Can you work these out from the model? Positions are in its coordinate system, mm. A direction names the side the tool comes from. Round coordinates to 2 decimals unless told otherwise and drop trailing zeros. Loops run counter-clockwise (first coordinate to the right, second up) from the corner with the lowest first, then second, coordinate; pieces in that order, holes last. Notation, with made-up numbers: M -22,35 L 35,35 A10 cw 35,41 Z; hole C 74.25,-31.75 d11. An arc over 180 degrees is marked long. Use a Markdown table: item, result. Add a question column.
Autodesk Fusion 360 part; units mm, degrees
sketch "Sketch1" plane through (0, 0, 0) normal (0, 0, 1) x (1, 0, 0)
  line L0 (-25, 25) -> (25, 25) construction
  line L1 (25, 25) -> (25, -25) construction
  line L2 (25, -25) -> (-25, -25) construction
  line L3 (-25, -25) -> (-25, 25) construction
  line L4 (-25, 25) -> (25, -25) construction
  line L5 (25, 25) -> (-25, -25) construction
  line L6 (24, 24) -> (-24, 24) construction
  line L7 (-24, 24) -> (-24, -24) construction
  line L8 (-24, -24) -> (24, -24) construction
  line L9 (24, -24) -> (24, 24) construction
  line L10 (24, 24) -> (-24, -24) construction
  line L11 (-24, 24) -> (24, -24) construction
  circle A0 centre (-22.5, 22.5) radius 1.5
  line L12 (0, 24) -> (0, -24)
  line L13 (-24, 0) -> (24, 0)
  circle A1 centre (-22.5, 22.5) radius 2.5 construction
  line L14 (-25, 0) -> (-25, 22.5)
  line L15 (0, 25) -> (-22.5, 25)
  arc A2 (-22.5, 25) -> (-25, 22.5) centre (-22.5, 22.5) ccw
  circle A3 centre (22.5, 22.5) radius 1.5
  arc A4 (25, 22.5) -> (22.5, 25) centre (22.5, 22.5) ccw
  line L16 (25, 0) -> (25, 22.5)
  line L17 (0, 25) -> (22.5, 25)
  circle A5 centre (-22.5, -22.5) radius 1.5
  arc A6 (-25, -22.5) -> (-22.5, -25) centre (-22.5, -22.5) ccw
  arc A7 (22.5, -25) -> (25, -22.5) centre (22.5, -22.5) ccw
  line L18 (25, 0) -> (25, -22.5)
  line L19 (0, -25) -> (-22.5, -25)
  line L20 (0, -25) -> (22.5, -25)
  line L21 (-25, 0) -> (-25, -22.5)
  circle A8 centre (22.5, -22.5) radius 1.5
  dimension "d1" = 50
  dimension "d2" = 50
  dimension "d3" = 48
  dimension "d4" = 48
  dimension "d5" = 1.5
extrude "Extrude1" add sketch "Sketch1" along normal blind 3
sketch "Sketch2" plane through (0, 0, 3) normal (0, 0, 1) x (-1, 0, 0)
  circle A0 centre (22.5, -22.5) radius 1.5
  circle A1 centre (-22.5, -22.5) radius 1.5
  circle A2 centre (-22.5, 22.5) radius 1.5
  circle A3 centre (22.5, 22.5) radius 1.5
  line L0 (-22.5, -25) -> (22.5, -25)
  arc A4 (22.5, -25) -> (25, -22.5) centre (22.5, -22.5) ccw
  line L1 (25, -22.5) -> (25, 22.5)
  arc A5 (25, 22.5) -> (22.5, 25) centre (22.5, 22.5) ccw
  line L2 (22.5, 25) -> (-22.5, 25)
  arc A6 (-22.5, 25) -> (-25, 22.5) centre (-22.5, 22.5) ccw
  line L3 (-25, 22.5) -> (-25, -22.5)
  arc A7 (-25, -22.5) -> (-22.5, -25) centre (-22.5, -22.5) ccw
  line L4 (18, 20) -> (10, 20)
  line L5 (10, 20) -> (10, 27)
  line L6 (10, 27) -> (18, 27)
  line L7 (18, 27) -> (18, 20)
  line L8 (8.1443, 19.89) -> (1.4935, 19.89)
  line L9 (1.4935, 19.89) -> (1.4935, 25)
  line L10 (1.4935, 25) -> (8.1443, 25)
  line L11 (8.1443, 25) -> (8.1443, 19.89)
  line L12 (-6.1327, 6.202) -> (-13.0241, 6.202)
  line L13 (-13.0241, 6.202) -> (-13.0241, 13.2304)
  line L14 (-13.0241, 13.2304) -> (-6.1327, 13.2304)
  line L15 (-6.1327, 13.2304) -> (-6.1327, 6.202)
  line L16 (9.0194, 12.5915) -> (1.9406, 12.5915)
  line L17 (1.9406, 12.5915) -> (1.9406, 3.3668)
  line L18 (1.9406, 3.3668) -> (9.0194, 3.3668)
  line L19 (9.0194, 3.3668) -> (9.0194, 12.5915)
  line L20 (18.1054, 2.8016) -> (12.2514, 2.8016)
  line L21 (12.2514, 2.8016) -> (12.2514, 8.8879)
  line L22 (12.2514, 8.8879) -> (18.1054, 8.8879)
  line L23 (18.1054, 8.8879) -> (18.1054, 2.8016)
  line L24 (23.1634, -18.1139) -> (7.6017, -18.1139)
  line L25 (7.6017, -18.1139) -> (7.6017, -12.2414)
  line L26 (7.6017, -12.2414) -> (23.1634, -12.2414)
  line L27 (23.1634, -12.2414) -> (23.1634, -18.1139)
  line L28 (-1.1153, -18.1139) -> (-17.3248, -18.1139)
  line L29 (-17.3248, -18.1139) -> (-17.3248, -12.2845)
  line L30 (-17.3248, -12.2845) -> (-1.1153, -12.2845)
  line L31 (-1.1153, -12.2845) -> (-1.1153, -18.1139)
  line L32 (17.5, -21) -> (9.5, -21)
  line L33 (9.5, -21) -> (9.5, -29)
  line L34 (9.5, -29) -> (17.5, -29)
  line L35 (17.5, -29) -> (17.5, -21)
  line L36 (-4, -21) -> (-12, -21)
  line L37 (-12, -21) -> (-12, -29)
  line L38 (-12, -29) -> (-4, -29)
  line L39 (-4, -29) -> (-4, -21)
  line L40 (-21.1194, -13.1989) -> (-25, -13.1989)
  line L41 (-25, -13.1989) -> (-25, -6.7401)
  line L42 (-25, -6.7401) -> (-21.1194, -6.7401)
  line L43 (-21.1194, -6.7401) -> (-21.1194, -13.1989)
  line L44 (-17, -0.5) -> (-33, -0.5)
  line L45 (-33, -0.5) -> (-33, 5.5)
  line L46 (-33, 5.5) -> (-17, 5.5)
  line L47 (-17, 5.5) -> (-17, -0.5)
  dimension "d8" = 2
  dimension "d9" = 7
  dimension "d10" = 8
  dimension "d11" = 7
  dimension "d12" = 4
  dimension "d13" = 8
  dimension "d14" = 8
  dimension "d15" = 8
  dimension "d16" = 7.5
  dimension "d17" = 13
  dimension "d18" = 8
  dimension "d19" = 6
  dimension "d20" = 16
  dimension "d21" = 19.5
extrude "Extrude2" add sketch "Sketch2" along normal blind 8 contours L3 L44 L45 L46 | L3 L44 L46 L47
extrude "Extrude3" add sketch "Sketch2" along normal blind 5 contours L0 L36 L37 L39 | L0 L37 L38 L39 | L0 L32 L33 L35 | L0 L33 L34 L35
extrude "Extrude4" add sketch "Sketch2" along normal blind 3 contours L3 L40 L41 L42 L43 | L2 L8 L9 L10 L11 | L2 L4 L5 L7 | L2 L5 L6 L7
extrude "Extrude5" add sketch "Sketch2" along normal blind 2 contours L16 L17 L18 L19
extrude "Extrude6" add sketch "Sketch2" along normal blind 1.5 contours L12 L13 L14 L15 | L20 L21 L22 L23 | L24 L25 L26 L27 | L28 L29 L30 L31
sketch "Sketch3" plane through (0, 0, 3) normal (0, 0, 1) x (-1, 0, 0)
  line L0 (-1.1153, -12.2845) -> (-1.1153, -18.1139)
  line L1 (-1.1153, -18.1139) -> (-17.3248, -18.1139)
  line L2 (-17.3248, -18.1139) -> (-17.3248, -12.2845)
  line L3 (-17.3248, -12.2845) -> (-1.1153, -12.2845)
  line L4 (-6.1327, 13.2304) -> (-6.1327, 6.202)
  line L5 (-6.1327, 6.202) -> (-13.0241, 6.202)
  line L6 (-13.0241, 6.202) -> (-13.0241, 13.2304)
  line L7 (-13.0241, 13.2304) -> (-6.1327, 13.2304)
  line L8 (23.1634, -12.2414) -> (23.1634, -18.1139)
  line L9 (23.1634, -18.1139) -> (7.6017, -18.1139)
  line L10 (7.6017, -18.1139) -> (7.6017, -12.2414)
  line L11 (7.6017, -12.2414) -> (23.1634, -12.2414)
  line L12 (18.1054, 8.8879) -> (18.1054, 2.8016)
  line L13 (18.1054, 2.8016) -> (12.2514, 2.8016)
  line L14 (12.2514, 2.8016) -> (12.2514, 8.8879)
  line L15 (12.2514, 8.8879) -> (18.1054, 8.8879)
  line L16 (9.0194, 3.3668) -> (1.9406, 3.3668)
  line L17 (1.9406, 3.3668) -> (1.9406, 12.5915)
  line L18 (1.9406, 12.5915) -> (9.0194, 12.5915)
  line L19 (9.0194, 12.5915) -> (9.0194, 3.3668)
  line L20 (-21.1194, -13.1989) -> (-25, -13.1989)
  line L21 (-25, -13.1989) -> (-25, -22.5)
  arc A0 (-25, -22.5) -> (-22.5, -25) centre (-22.5, -22.5) ccw
  line L22 (-22.5, -25) -> (-12, -25)
  line L23 (-12, -25) -> (-12, -21)
  line L24 (-12, -21) -> (-4, -21)
  line L25 (-4, -21) -> (-4, -25)
  line L26 (-4, -25) -> (9.5, -25)
  line L27 (9.5, -25) -> (9.5, -21)
  line L28 (9.5, -21) -> (17.5, -21)
  line L29 (17.5, -21) -> (17.5, -25)
  line L30 (17.5, -25) -> (22.5, -25)
  arc A1 (22.5, -25) -> (25, -22.5) centre (22.5, -22.5) ccw
  line L31 (25, -22.5) -> (25, 22.5)
  arc A2 (25, 22.5) -> (22.5, 25) centre (22.5, 22.5) ccw
  line L32 (22.5, 25) -> (18, 25)
  line L33 (18, 25) -> (18, 20)
  line L34 (18, 20) -> (10, 20)
  line L35 (10, 20) -> (10, 25)
  line L36 (10, 25) -> (8.1443, 25)
  line L37 (8.1443, 25) -> (8.1443, 19.89)
  line L38 (8.1443, 19.89) -> (1.4935, 19.89)
  line L39 (1.4935, 19.89) -> (1.4935, 25)
  line L40 (1.4935, 25) -> (-22.5, 25)
  arc A3 (-22.5, 25) -> (-25, 22.5) centre (-22.5, 22.5) ccw
  line L41 (-25, 22.5) -> (-25, 5.5)
  line L42 (-25, 5.5) -> (-17, 5.5)
  line L43 (-17, 5.5) -> (-17, -0.5)
  line L44 (-17, -0.5) -> (-25, -0.5)
  line L45 (-25, -0.5) -> (-25, -6.7401)
  line L46 (-25, -6.7401) -> (-21.1194, -6.7401)
  line L47 (-21.1194, -6.7401) -> (-21.1194, -13.1989)
  circle A4 centre (22.5, -22.5) radius 1.5
  circle A5 centre (-22.5, -22.5) radius 1.5
  circle A6 centre (-22.5, 22.5) radius 1.5
  circle A7 centre (22.5, 22.5) radius 1.5
  line L48 (4.6554, 14.7653) -> (3.1888, 14.7653)
  line L49 (3.1888, 14.7653) -> (3.1888, 15.6382)
  line L50 (3.1888, 15.6382) -> (4.6554, 15.6382)
  line L51 (4.6554, 15.6382) -> (4.6554, 14.7653)
  line L52 (4.6554, 16.2319) -> (3.1888, 16.2319)
  line L53 (3.1888, 16.2319) -> (3.1888, 17.2096)
  line L54 (3.1888, 17.2096) -> (4.6554, 17.2096)
  line L55 (4.6554, 17.2096) -> (4.6554, 16.2319)
extrude "Extrude7" add sketch "Sketch3" along normal blind 0.1 contours L48 L49 L50 L51 | L52 L53 L54 L55
equation "d15 = d14"
(1) I'm going to push flat-ended pins straight in: pin 1 (5.5 mm diameter, centred on x = -4.5, y = -21.5, fed in from +Z); pin 2 (1.2 mm diameter, centred on y = -8, z = 4, fed in from +X); pin 3 (0.9 mm diameter, centred on y = 9.5, z = 5, fed in from -X); pin 4 (1.5 mm diameter, centred on y = 20, z = 5.5, fed in from +X). Where does each tip first touch, or does it pass through?
(2) If I drill on probe 1 along Y at (x, z) = (22.5, 2.3); probe 2 along Z at (x, y) = (-10.5, 23); probe 3 along Z at (x, y) = (-11, 27), over which ranges is the centre line in solid material (lowest first)? Write a range as [from, to].
(3) Suppose I cut it at C-C on z = 9.75. List the corners of the cut face in (x, y) for me.
(4) Thinking about a two-plate mould opening in X: for faces 4 (the face through (8, 27, 3)), 5 (the face through (-18.105, -6, 4)), 6 (the face through (-23.61, -23.51, 1.48)), which applies, released by +X, released by -X, zero draft, split by the parting line, or undercut?
(5) On a 3-axis mill with a long thin cutter (end or side, diameter ignored), from which of +Z, -Z, +X, -X, +Y, -Y can I reach the whole of each face in a straight line? I mean faces 1 (the face through (1.115, 15, 4)), 2 (the face through (-14, -20, 4)), 3 (the face through (-10, -23, 4)). Say none if no direction works.
(6) Suppose I cut it at B-B on y = 6. List the corners of the cut face in (x, z) for me.
(7) Suppose I cut it at A-A on x = 15.5. List the corners of the cut face in (y, z) for me.
Results below:
| question | item | result |
|---|---|---|
| 1 | pin 1 | stops at z = 6 |
| 1 | pin 2 | stops at x = 13.02 |
| 1 | pin 3 | stops at x = 21.12 |
| 1 | pin 4 | passes through |
| 2 | probe 1 | y = [-25, -24], [-21, 21], [24, 25] |
| 2 | probe 2 | z = [0, 8] |
| 2 | probe 3 | z = [3, 8] |
| 3 | outline | M 17,-5.5 L 33,-5.5 L 33,0.5 L 17,0.5 Z |
| 4 | face 4 | zero draft |
| 4 | face 5 | released by -X |
| 4 | face 6 | undercut |
| 5 | face 1 | +Z, +Y, -Y |
| 5 | face 2 | +Z, -X |
| 5 | face 3 | +Z, -Y |
| 6 | outline | M -25,0 L 25,0 L 25,3 L -25,3 Z |
| 7 | outline | M -25,0 L 25,0 L 25,3 L 18.11,3 L 18.11,4.5 L 12.28,4.5 L 12.28,3 L -25,3 Z |
